Design review of the part built by this model. Coordinates are the model's own, in mm. Face numbers are marked on the shaded views. A direction names the side the tool comes from. Coordinates: 2 decimals unless noted, no trailing zeros. Loops run counter-clockwise (first coordinate to the right, second up) from the corner with the lowest first, then second, coordinate; pieces in that order, holes last. Notation, with made-up numbers: M 50.5,22.25 L 102.5,22.25 A25 cw 102.5,51.25 Z; hole C 19.25,21 d5. An arc over 180 degrees is marked long. Answer as a JSON object with one key per item and string values. Group by question number.
1. To check wall thickness, follow probe 1 along Z at (x, y) = (-50.8, 9.75); probe 2 along Y at (x, z) = (-25, -1.5); probe 3 along X at (y, z) = (-9, 5.25) (3 decimals). State the ranges of each line that lie inside material, in increasing order.
2. Consider section C-C (z = 5). State the section outline as (x, y) points (3 decimals), then the cut area to 3 significant figures.
3. Consider section A-A (x = -50.8). State the section outline as (y, z) points, then the cut area to 3 significant figures.
4. Machinability: for the marked faces 1, 2 and 3, which of the approach directions +Z, -Z, +X, -X, +Y, -Y give a long, thin tool a straight path to every point of the face, cutting with its end or side? Answer none if there is none.
5. Insertion check: pin 1 (5 mm diameter, centred on y = -15, z = 2.5, fed in from +X) (3 decimals); pin 2 (10 mm diameter, centred on x = 44, z = 7.5, fed in from -Y); pin 3 (6 mm diameter, centred on x = -1.5, z = -8, fed in from -Y). Each pin has a flat end and moves straight along its axis. Give the tip position at first contact, or say it passes through.
6. Consider section D-D (y = -7.5). State the section outline as (x, z) points (3 decimals).
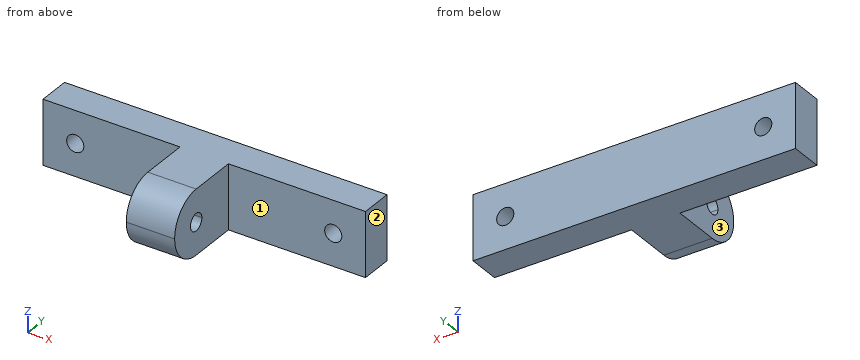
from build123d import *

# Parameters (mm, degrees)
SKETCH1_W           = 19.05
SKETCH1_H           = 12.7
BOSS_EXTRUDE1_DEPTH = 12.7
SKETCH1_3_W         = 19.05
SKETCH1_3_H         = 12.7
BOSS_EXTRUDE2_DEPTH = 31.75
CUT_EXTRUDE1_DEPTH  = 81.63499938
FILLET1_R           = 12.7


with BuildPart() as part:
    # Sketch1 → Boss-Extrude1 (new body)
    with BuildSketch(Plane(origin=(0, 0, 0), x_dir=(1, 0, 0), z_dir=(0, 1, 0))):
        with BuildLine():
            Line((63.5, 12.7), (9.525, 12.7))
            Line((9.525, 12.7), (9.525, 0))
            Line((9.525, 0), (47.4218, 0))
            ThreePointArc((47.4218, 0), (50.8, 3.3782), (54.1782, 0))
            Line((54.1782, 0), (63.5, 0))
            Line((63.5, 0), (63.5, 12.7))
        make_face()
        with BuildLine():
            Line((47.4218, 0), (9.525, 0))
            Line((9.525, 0), (9.525, -12.7))
            Line((9.525, -12.7), (63.5, -12.7))
            Line((63.5, -12.7), (63.5, 0))
            Line((63.5, 0), (54.1782, 0))
            ThreePointArc((54.1782, 0), (50.8, -3.3782), (47.4218, 0))
        make_face()
        with Locations((0, -6.35)):
            Rectangle(SKETCH1_W, SKETCH1_H)
        with Locations((0, 6.35)):
            Rectangle(SKETCH1_W, SKETCH1_H)
        with BuildLine():
            Line((-54.1782, 0), (-63.5, 0))
            Line((-63.5, 0), (-63.5, -12.7))
            Line((-63.5, -12.7), (-9.525, -12.7))
            Line((-9.525, -12.7), (-9.525, 0))
            Line((-9.525, 0), (-47.4218, 0))
            ThreePointArc((-47.4218, 0), (-50.8, -3.3782), (-54.1782, 0))
        make_face()
        with BuildLine():
            Line((-9.525, 12.7), (-63.5, 12.7))
            Line((-63.5, 12.7), (-63.5, 0))
            Line((-63.5, 0), (-54.1782, 0))
            ThreePointArc((-54.1782, 0), (-50.8, 3.3782), (-47.4218, 0))
            Line((-47.4218, 0), (-9.525, 0))
            Line((-9.525, 0), (-9.525, 12.7))
        make_face()
    extrude(amount=BOSS_EXTRUDE1_DEPTH)

    # Sketch1<3> → Boss-Extrude2 (add)
    with BuildSketch(Plane(origin=(0, 0, 0), x_dir=(1, 0, 0), z_dir=(0, 1, 0))):
        with Locations((0, -6.35)):
            Rectangle(SKETCH1_3_W, SKETCH1_3_H)
        with Locations((0, 6.35)):
            Rectangle(SKETCH1_3_W, SKETCH1_3_H)
    extrude(amount=-BOSS_EXTRUDE2_DEPTH)

    # Sketch2 → Cut-Extrude1 (cut, through all)
    with BuildSketch(Plane.ZY.offset(9.525)):
        with BuildLine():
            ThreePointArc((3.3782, -19.05), (2.388748128, -16.661251872), (0, -15.6718))
            Line((0, -15.6718), (0, -22.4282))
            ThreePointArc((0, -22.4282), (2.388748128, -21.438748128), (3.3782, -19.05))
        make_face()
        with BuildLine():
            Line((0, -22.4282), (0, -15.6718))
            ThreePointArc((0, -15.6718), (-3.3782, -19.05), (0, -22.4282))
        make_face()
    extrude(amount=-CUT_EXTRUDE1_DEPTH, mode=Mode.SUBTRACT)

    # Fillet1
    fillet1_edges = [part.edges().sort_by_distance(p)[0] for p in [
        (0, -31.75, -12.7),
        (0, -31.75, 12.7),
    ]]
    fillet(fillet1_edges, radius=FILLET1_R - 0.0001)  # a hair under: the kernel refuses the full size


solid = part.part
Findings below:
{
 "1": {"probe 1": "z = -12.7 to -3.38, 3.38 to 12.7", "probe 2": "y = 0 to 12.7", "probe 3": "x = -9.525 to 9.525"},
 "2": {"outline": "M -63.5,0 L -9.525,0 L -9.525,-30.724 L 9.525,-30.724 L 9.525,0 L 63.5,0 L 63.5,12.7 L -63.5,12.7 Z", "area": "2,200 mm^2"},
 "3": {"outline": "M 0,-12.7 L 12.7,-12.7 L 12.7,-3.38 L 0,-3.38 Z; M 0,3.38 L 12.7,3.38 L 12.7,12.7 L 0,12.7 Z", "area": "237 mm^2"},
 "4": {"face 1": "+Z, -Z, +X, -Y", "face 2": "+Z, -Z, +X, +Y, -Y", "face 3": "+Z, -Z, -X, -Y"},
 "5": {"pin 1": "stops at x = 9.525", "pin 2": "stops at y = 0", "pin 3": "stops at y = -30.72"},
 "6": {"outline": "M -9.525,-12.7 L 9.525,-12.7 L 9.525,12.7 L -9.525,12.7 Z"}
}
